Model file for the job. Use its own axes, mm. A direction names the side the tool comes from. Round coordinates to 2 decimals unless told otherwise and drop trailing zeros. Write each loop counter-clockwise with the first axis right and the second up, starting at its lowest first coordinate (ties: lowest second). Pieces come first, ordered by that corner, then holes. Notation, with made-up numbers: (20.25, -18.75) - (46.25, -18.75) arc R17 cw to (46.25, -10.75) - close; hole circle Ø5 at (55, 4.5). An arc over 180 degrees is marked (long way). Answer as a JSON object with one key per item and string values. Group by question number.
from build123d import *

# Parameters (mm, degrees)
BOSS_EXTRU_2_DEPTH      = 19
ESQUISSE3_R             = 2.5
ENL_V_MAT_EXTRU_1_DEPTH = 81.564305533
ENL_V_MAT_EXTRU_2_DEPTH = 3
CHANFREIN1_SIZE         = 4
ESQUISSE7_W             = 7
ESQUISSE7_H             = 50
ENL_V_MAT_EXTRU_4_DEPTH = 19
BOSS_EXTRU_3_REACH      = 82.564
ENL_V_START             = 6
ENL_V_MAT_EXTRU_7_DEPTH = 6
CONG_2_R                = 2
CHANFREIN2_SIZE         = 1
ESQUISSE9_R             = 2.25
ENL_V_MAT_EXTRU_5_DEPTH = 81.564305533


with BuildPart() as part:
    # Esquisse1 → Boss.-Extru.2 (new body)
    with BuildSketch(Plane(origin=(0, 20, 0), x_dir=(1, 0, 0), z_dir=(0, 1, 0))):
        with BuildLine():
            Line((25.673562069, 38.419058892), (25.673562069, -16.580941108))
            ThreePointArc((25.673562069, -16.580941108), (25.974401889, -18.535528805), (26.849073781, -20.309187945))
            Line((26.849073781, -20.309187945), (46.924249054, -48.979509495))
            ThreePointArc((46.924249054, -48.979509495), (55.976984178, -50.575750946), (57.573225629, -41.523015822))
            Line((57.573225629, -41.523015822), (39.758649804, -16.081164865))
            ThreePointArc((39.758649804, -16.081164865), (38.951260365, -14.443941044), (38.673562069, -12.639706247))
            Line((38.673562069, -12.639706247), (38.673562069, 38.419058892))
            Line((38.673562069, 38.419058892), (25.673562069, 38.419058892))
        make_face()
    extrude(amount=BOSS_EXTRU_2_DEPTH)

    # Esquisse3 → Enlèv. mat.-Extru.1 (cut, through all)
    with BuildSketch(Plane(origin=(0, 39, 0), x_dir=(1, 0, 0), z_dir=(0, 1, 0))):
        with Locations(Location((32.173562069, -16.580941108, 0), (0, 0, 270))):
            Circle(ESQUISSE3_R)
        with Locations(Location((52.248737342, -45.251262658, 0), (0, 0, 270))):
            Circle(ESQUISSE3_R)
    extrude(amount=-ENL_V_MAT_EXTRU_1_DEPTH, mode=Mode.SUBTRACT)

    # Esquisse4 → Enlèv. mat.-Extru.2 (cut, symmetric)
    with BuildSketch(Plane(origin=(0, 29.5, 0), x_dir=(1, 0, 0), z_dir=(0, 1, 0))):
        with BuildLine():
            Line((57.573225629, -41.523015822), (51.26388483, -32.512343335))
            Line((51.26388483, -32.512343335), (40.614908254, -39.968837008))
            Line((40.614908254, -39.968837008), (46.924249054, -48.979509495))
            ThreePointArc((46.924249054, -48.979509495), (55.976984178, -50.575750946), (57.573225629, -41.523015822))
        make_face()
    extrude(amount=ENL_V_MAT_EXTRU_2_DEPTH, both=True, mode=Mode.SUBTRACT)

    # Chanfrein1
    chanfrein1_edges = [part.edges().sort_by_distance(p)[0] for p in [
        (40.614908254, 29.5, 39.968837008),
    ]]
    chamfer(chanfrein1_edges, length=CHANFREIN1_SIZE)

    # Esquisse7 → Enlèv. mat.-Extru.4 (cut)
    with BuildSketch(Plane(origin=(0, 39, 0), x_dir=(1, 0, 0), z_dir=(0, 1, 0))):
        with Locations((29.173562069, 13.419058892)):
            Rectangle(ESQUISSE7_W, ESQUISSE7_H)
    extrude(amount=-ENL_V_MAT_EXTRU_4_DEPTH, mode=Mode.SUBTRACT)

    # Boss.-Extru.3: up to this face of the body (flat: up to its plane)
    boss_extru_3_end = Plane(part.part.faces().sort_by_distance((29.173562069, 20, 12.541391737))[0])
    # Esquisse8 → Boss.-Extru.3 (add, up to the picked face)
    with BuildSketch(Plane(origin=(0, 39, 0), x_dir=(1, 0, 0), z_dir=(0, 1, 0)), mode=Mode.PRIVATE) as boss_extru_3_sk1:
        with BuildLine():
            Line((38.673562069, 38.419058892), (41.673562069, 38.419058892))
            Line((41.673562069, 38.419058892), (58.615433045, -43.941611626))
            Line((58.615433045, -43.941611626), (57.573225629, -43.941611626))
            Line((57.573225629, -43.941611626), (57.573225629, -41.523015822))
            Line((57.573225629, -41.523015822), (39.758649804, -16.081164865))
            ThreePointArc((39.758649804, -16.081164865), (38.951260365, -14.443941044), (38.673562069, -12.639706247))
            Line((38.673562069, -12.639706247), (38.673562069, 38.419058892))
        make_face()
    boss_extru_3_tool1 = split(extrude(boss_extru_3_sk1.sketch, amount=-BOSS_EXTRU_3_REACH, mode=Mode.PRIVATE), bisect_by=boss_extru_3_end, keep=Keep.BOTH, mode=Mode.PRIVATE)
    add(boss_extru_3_tool1.solids().sort_by(Axis((45.454981, 39, 2.99996), (0, -1, 0)))[0])

    # Esquisse11 → Enlèv. mat.-Extru.7 (cut)
    with BuildSketch(Plane.XZ.offset(-32.5).offset(ENL_V_START)):
        with BuildLine():
            Line((51.26388483, 32.512343335), (43.891516431, 37.674531262))
            Line((43.891516431, 37.674531262), (38.320602508, 36.69222883))
            Line((38.320602508, 36.69222883), (46.924249054, 48.979509495))
            ThreePointArc((46.924249054, 48.979509495), (54.821022864, 51.220630062), (58.615433045, 43.941611626))
            Line((58.615433045, 43.941611626), (55.634824859, 29.451778178))
            Line((55.634824859, 29.451778178), (51.26388483, 32.512343335))
        make_face()
    extrude(amount=-ENL_V_MAT_EXTRU_7_DEPTH, mode=Mode.SUBTRACT)

    # Congé2
    cong_2_edges = [part.edges().sort_by_distance(p)[0] for p in [
        (25.673562069, 29.5, 11.580941108),
    ]]
    fillet(cong_2_edges, radius=CONG_2_R)

    # Chanfrein2
    chanfrein2_edges = [part.edges().sort_by_distance(p)[0] for p in [
        (32.673562069, 29.5, -38.419058892),
    ]]
    chamfer(chanfrein2_edges, length=CHANFREIN2_SIZE)

    # Esquisse9 → Enlèv. mat.-Extru.5 (cut, through all)
    with BuildSketch(Plane(origin=(0, 39, 0), x_dir=(1, 0, 0), z_dir=(0, 1, 0))):
        with Locations(Location((38.423562069, 23.419058892, 0), (0, 0, 270))):
            Circle(ESQUISSE9_R)
        with Locations(Location((38.423562069, -1.580941108, 0), (0, 0, 270))):
            Circle(ESQUISSE9_R)
    extrude(amount=-ENL_V_MAT_EXTRU_5_DEPTH, mode=Mode.SUBTRACT)


solid = part.part
(1) 3-axis set-ups, long thin cutter, end or side, ignore diameter. For faces 5 (the cylindrical face through (37.05, 29.63, -25.2)), 6 (the flat face through (41.15, 29.46, 37.19)), 7 (the flat face through (30, 30, 11.581)): which of +Z, -Z, +X, -X, +Y, -Y reach the whole face in a straight line?
(2) Slice it at D-D (y = 34.25). Write the cut outline in (x, z).
(3) Flat gauge pins, fed straight in: pin 1 (8 mm diameter, centred on y = 27, z = 38.5, fed in from -X); pin 2 (4 mm diameter, centred on x = 30.5, y = 27.5, fed in from -Z); pin 3 (5 mm diameter, centred on x = 34.5, y = 37, fed in from +Z). Where does each tip first touch, or does it go through?
(4) Slice it at A-A (z = 39). Write the cut outline in (x, y).
(5) Slice it at C-C (y = 29). Write the cut outline in (x, z).
(6) Slice it at B-B (x = 37.5). Write the cut outline in (y, z).
(7) Pull direction Z, two halves, no side cores. Call faces 1 (the cylindrical face through (26.244, 29.367, 12.182)), 2 (the cylindrical face through (51.29, 35.8, 47.56)), 3 (the cylindrical face through (36.227, 29.633, 1.093)), 4 (the flat face through (42, 39, 6)): pulls with the +Z half, pulls with the -Z half, needs draft (parallel to the pull), parting line crosses it, or undercut.
(8) Drill centre lines: line 1 (Y direction, x = 42.5, z = 40); line 2 (Z direction, x = 38.5, y = 26); line 3 (Z direction, x = 38, y = 21.25). Where is each one in solid material? Low to high. Write a range as from..to.
Answer:
{
 "1": {"face 5": "+Y, -Y", "face 6": "+Z, -X", "face 7": "-Z, -X, +Y, -Y"},
 "2": {"outline": "(25.67, 13.58) arc R2 ccw to (27.67, 11.58) - (32.67, 11.58) - (32.67, -37.42) - (33.67, -38.42) - (41.67, -38.42) - (58.62, 43.94) arc R6.5 ccw to (46.92, 48.98) - (26.85, 20.31) arc R6.5 ccw to (25.67, 16.58) - close; hole circle Ø5 at (32.17, 16.58); hole circle Ø4.5 at (38.42, -23.42); hole circle Ø4.5 at (38.42, 1.58); hole circle Ø5 at (52.25, 45.25)"},
 "3": {"pin 1": "x = 36.79", "pin 2": "z = 11.58", "pin 3": "z = 34.81"},
 "4": {"outline": "(39.94, 20) - (57.6, 20) - (57.6, 26.5) - (39.94, 26.5) - close; (39.94, 32.5) - (57.6, 32.5) - (57.6, 39) - (39.94, 39) - close"},
 "5": {"outline": "(25.67, 13.58) arc R2 ccw to (27.67, 11.58) - (32.67, 11.58) - (32.67, -37.42) - (33.67, -38.42) - (41.67, -38.42) - (55.63, 29.45) - (43.89, 37.67) - (38.32, 36.69) - (26.85, 20.31) arc R6.5 ccw to (25.67, 16.58) - close; hole circle Ø5 at (32.17, 16.58); hole circle Ø4.5 at (38.42, -23.42); hole circle Ø4.5 at (38.42, 1.58)"},
 "6": {"outline": "(20, -38.42) - (39, -38.42) - (39, -25.47) - (20, -25.47) - close; (20, -21.37) - (39, -21.37) - (39, -0.47) - (20, -0.47) - close; (20, 3.63) - (39, 3.63) - (39, 35.52) - (20, 35.52) - close"},
 "7": {"face 1": "pulls with the -Z half", "face 2": "undercut", "face 3": "undercut", "face 4": "needs draft"},
 "8": {"line 1": "20..26.5, 32.5..39", "line 2": "-38.42..-25.67, -21.17..-0.67, 3.83..36.95", "line 3": "-38.42..-25.63, -21.21..-0.63, 3.79..36.23"}
}
